Could you check a few things on this model? Use its own coordinates, in mm. A direction names the side the tool comes from. Give positions to 0.01 mm unless a question says otherwise; leave off trailing zeros. Order: outer loops, then holes, each group sorted by start corner. A loop starts at its lowest first (then second) coordinate and runs counter-clockwise, first axis right, second up. Notation, with made-up numbers: M -29.5,-2 L -8.5,-2 A30 ccw -8.5,31 Z; hole C 30.5,12.25 d3. An arc over 180 degrees is marked long. Use a Markdown table: item, result. Add a question column.
Item 1: Suppose I cut it at C-C on x = 0. Write out the boundary of the cut face in (y, z).
Item 2: If we mould it in two halves opening along X, with no side actions, what happens to faces 3 (the face through (93.96, -32.282, 14.79)), 4 (the face through (1.08, -4.88, 4.93)), 5 (the face through (84, 1, 0))? For each: released by +X, released by -X, zero draft, split by the parting line, or undercut.
Item 3: For faces 1 (the face through (0, 0, 10)), 2 (the face through (84, 1, 30)), which set-ups out of +Z, -Z, +X, -X, +Y, -Y let a thin tool reach every point of the face, with its end or its side?
Item 4: Suppose I cut it at D-D on z = 7. Write out the boundary of the cut face in (x, y).
Item 5: If I drill on L1, parallel to Y at x = 0, z = 1.5; L2, parallel to Y at x = 180, z = 14.25; L3, parallel to X at y = -3.5, z = 25, over which ranges is the centre line in solid material (lowest first)? Write a range as from..to.
Item 6: Suppose I cut it at A-A on y = 0. Write out the boundary of the cut face in (x, z), plus the area to 3 significant figures.
Item 7: I'm going to push flat-ended pins straight in: pin 1 Ø12 at (x, z) = (118.5, 26.5) entering from -Y; pin 2 Ø4 at (x, z) = (136, 25.5) entering from -Y; pin 3 Ø6 at (x, z) = (33.5, 12.5) entering from +Y. Where does each tip first touch, or does it pass through?
Item 8: Suppose I cut it at B-B on z = 18. Write out the boundary of the cut face in (x, y), plus the area to 3 significant figures.
from build123d import *

# Parameters (mm, degrees)
BOSS_EXTRUDE1_DEPTH = 30
SKETCH2_R           = 5
CUT_EXTRUDE1_DEPTH  = 10
SKETCH3_R           = 7.5
CUT_EXTRUDE2_DEPTH  = 69


with BuildPart() as part:
    # Sketch1 → Boss-Extrude1 (new body)
    with BuildSketch(Plane.XY):
        with BuildLine():
            Line((3.333333333, 39.860869144), (182.083333333, 24.913043215))
            ThreePointArc((182.083333333, 24.913043215), (205, 0), (182.083333333, -24.913043215))
            Line((182.083333333, -24.913043215), (3.333333333, -39.860869144))
            ThreePointArc((3.333333333, -39.860869144), (-40, 0), (3.333333333, 39.860869144))
        make_face()
    extrude(amount=BOSS_EXTRUDE1_DEPTH)

    # Sketch2 → Cut-Extrude1 (cut)
    with BuildSketch(Plane(origin=(0, 0, 0), x_dir=(-1, 0, 0), z_dir=(0, 0, -1))):
        Circle(SKETCH2_R)
    extrude(amount=-CUT_EXTRUDE1_DEPTH, mode=Mode.SUBTRACT)

    # Sketch3 → Cut-Extrude2 (cut)
    with BuildSketch(Plane.XY.offset(30)):
        with Locations((180, 0)):
            Circle(SKETCH3_R)
    extrude(amount=-CUT_EXTRUDE2_DEPTH, mode=Mode.SUBTRACT)


solid = part.part
Findings below:
| question | item | result |
|---|---|---|
| 1 | outline | M -40,0 L -5,0 L -5,10 L 5,10 L 5,0 L 40,0 L 40,30 L -40,30 Z |
| 2 | face 3 | released by +X |
| 2 | face 4 | undercut |
| 2 | face 5 | zero draft |
| 3 | face 1 | -Z |
| 3 | face 2 | +Z, +X, -X, +Y, -Y |
| 4 | outline | M 3.33,-39.86 L 182.08,-24.91 A25 ccw 182.08,24.91 L 3.33,39.86 A40 ccw long Z; hole C 0,0 d10; hole C 180,0 d15 |
| 5 | L1 | y = -40..-5, 5..40 |
| 5 | L2 | y = -25.09..-7.5, 7.5..25.09 |
| 5 | L3 | x = -39.85..173.37, 186.63..204.75 |
| 6 | outline | M -40,0 L -5,0 L -5,10 L 5,10 L 5,0 L 172.5,0 L 172.5,30 L -40,30 Z; M 187.5,0 L 205,0 L 205,30 L 187.5,30 Z |
| 6 | area | 6,800 mm^2 |
| 7 | pin 1 | stops at y = -30.73 |
| 7 | pin 2 | stops at y = -28.93 |
| 7 | pin 3 | stops at y = 37.59 |
| 8 | outline | M 3.33,-39.86 L 182.08,-24.91 A25 ccw 182.08,24.91 L 3.33,39.86 A40 ccw long Z; hole C 180,0 d15 |
| 8 | area | 15,100 mm^2 |
